Verification items for the finished model (mm, model axes). Coordinates: 2 decimals unless noted, no trailing zeros. Loops run counter-clockwise (first coordinate to the right, second up) from the corner with the lowest first, then second, coordinate; pieces in that order, holes last.
Q1. Material ranges on probe 1 along Y at (x, z) = (-16.5, 20); probe 2 along X at (y, z) = (-3.5, 0); probe 3 along X at (y, z) = (-1, 2), recorded low to high.
Q2. Sectioned sample at B-B (x = -16.5). Enter the section's corners in (y, z).
Q3. Sectioned sample at A-A (z = -19.5). Enter the section's corners in (x, y).
Q4. Go/stop test with flat-tipped pins: P1, Ø2, axis at y = -1.5, z = 8, coming from the +X side; P2, Ø2, axis at y = -2, z = -17.5, coming from the -X side; P3, Ø1.5, axis at y = -4.5, z = -10.5, coming from the -X side. Record where each tip stops, or that it passes through.
```python
from build123d import *

# Parameters (mm, degrees)
F0_R     = 30
F1_DEPTH = 5
F4_DEPTH = 5
F5_DEPTH = 5
F6_DEPTH = 5
F7_DEPTH = 2


with BuildPart() as f1:
    # F0 (on Front) → F1 (new body)
    with BuildSketch(Plane.XZ):
        Circle(F0_R)
    extrude(amount=F1_DEPTH)

    # F3 (on face) → F4 (cut)
    with BuildSketch(Plane.XZ.offset(5)):
        with BuildLine():
            Line((-10.9299741999, 23.5023200512), (-5.5388955, 29.4842438709))
            ThreePointArc((-5.5388955, 29.4842438709), (-10.0449779303, 28.2683288926), (-14.3079358656, 26.3682189627))
            add(Edge.make_bspline(
                [(-14.3079358656, 26.3682189627), (-13.1550391421, 25.4607855158), (-12.0252922437, 24.5080470289), (-10.9299741999, 23.5023200512)],
                knots=[0, 0, 0, 0, 4.6870131966, 4.6870131966, 4.6870131966, 4.6870131966], degree=3))
        make_face()
    extrude(amount=-F4_DEPTH, mode=Mode.SUBTRACT)

    # F3 (on face) → F5 (cut)
    with BuildSketch(Plane.XZ.offset(5)):
        with BuildLine():
            Line((-17.9465766996, 17.9648566991), (-14.3079358656, 26.3682189627))
            ThreePointArc((-14.3079358656, 26.3682189627), (-18.3884401049, 23.7036974016), (-21.9836899596, 20.4136565995))
            add(Edge.make_bspline(
                [(-21.9836899596, 20.4136565995), (-20.642975191, 19.610865703), (-19.293517456, 18.7987052228), (-17.9465766996, 17.9648566991)],
                knots=[0, 0, 0, 0, 4.8486235733, 4.8486235733, 4.8486235733, 4.8486235733], degree=3))
        make_face()
    extrude(amount=-F5_DEPTH, mode=Mode.SUBTRACT)

    # F3 (on face) → F6 (cut)
    with BuildSketch(Plane.XZ.offset(5)):
        with BuildLine():
            Line((-23.1792298082, 11.114937143), (-21.9836899596, 20.4136565995))
            ThreePointArc((-21.9836899596, 20.4136565995), (-25.1493367192, 16.3557593094), (-27.5748147519, 11.8164965789))
            add(Edge.make_bspline(
                [(-27.5748147519, 11.8164965789), (-26.208679714, 11.6220681724), (-24.7320616466, 11.3922656282), (-23.1792298082, 11.114937143)],
                knots=[0, 0, 0, 0, 5.1239362549, 5.1239362549, 5.1239362549, 5.1239362549], degree=3))
        make_face()
    extrude(amount=-F6_DEPTH, mode=Mode.SUBTRACT)

    # F3 (on face) → F7 (join)
    with BuildSketch(Plane.XZ.offset(5)):
        with BuildLine():
            add(Edge.make_bspline(
                [(-5.5388955, 29.4842438709), (0, 23.5023200512), (4.6262064465, 13.365700841), (2.3032309004, 0)],
                knots=[0, 0, 0, 0, 30.5093359993, 30.5093359993, 30.5093359993, 30.5093359993], degree=3))
            Line((-5.5388955, 29.4842438709), (-10.9299741999, 23.5023200512))
            add(Edge.make_bspline(
                [(-10.9299741999, 23.5023200512), (-4.7424400597, 17.8208925919), (0.3463986774, 10.4484936531), (2.3032309004, 0)],
                knots=[4.6870131966, 4.6870131966, 4.6870131966, 4.6870131966, 31.1643038201, 31.1643038201, 31.1643038201, 31.1643038201], degree=3))
        make_face()
    extrude(amount=F7_DEPTH)


solid = f1.part
```
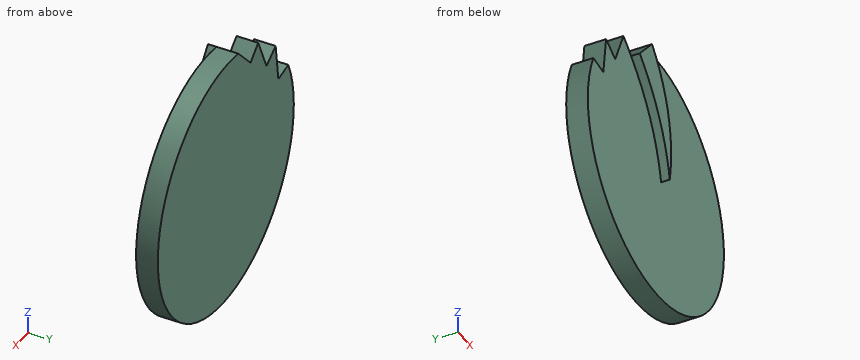
Geometry check:
1. probe 1: y = -5 to 0
1. probe 2: x = -30 to 30
1. probe 3: x = -29.93 to 29.93
2. outline: (-5, -25.05) - (0, -25.05) - (0, 21.31) - (-5, 21.31) - close
3. outline: (-22.8, -5) - (22.8, -5) - (22.8, 0) - (-22.8, 0) - close
4. P1: stops at x = 29.17
4. P2: stops at x = -25.05
4. P3: stops at x = -28.37
